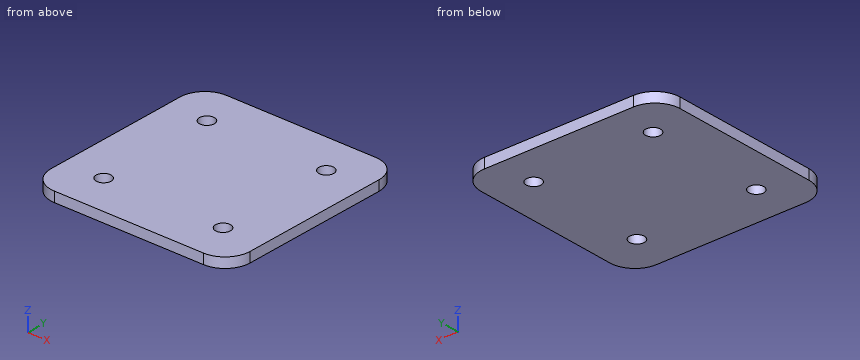
Autodesk Inventor part; units mm, degrees
ref_plane "YZ Plane" through (0, 0, 0) normal (1, 0, 0) x (0, 1, 0)
ref_plane "XZ Plane" through (0, 0, 0) normal (0, 1, 0) x (-1, 0, 0)
ref_plane "XY Plane" through (0, 0, 0) normal (0, 0, 1) x (1, 0, 0)
sketch "Sketch1" plane through (0, 0, 0) normal (0, 0, 1) x (1, 0, 0)
  line L0 (-20, -20) -> (20, -20)
  line L1 (20, -20) -> (20, 20)
  line L2 (20, 20) -> (-20, 20)
  line L3 (-20, 20) -> (-20, -20)
  line L4 (-20, -20) -> (20, 20) construction
  line L5 (20, -20) -> (-20, 20) construction
  line L6 (-12, -12) -> (12, -12) construction
  line L7 (12, -12) -> (12, 12) construction
  line L8 (12, 12) -> (-12, 12) construction
  line L9 (-12, 12) -> (-12, -12) construction
  line L10 (-12, -12) -> (12, 12) construction
  line L11 (12, -12) -> (-12, 12) construction
  point P0 (0, 0)
  dimension "d0" = 40
  dimension "d1" = 40
  dimension "d2" = 24
  dimension "d3" = 24
extrude "Extrusion1" add sketch "Sketch1" against normal blind 2
hole "Hole1" at (-12, 12, 0) at (12, 12, 0) at (12, -12, 0) at (-12, -12, 0) direction (0, 0, -1) diameter 3 depth 2
fillet "Fillet1" radius 5 4 edges at (20, 20, -1) (20, -20, -1) (-20, -20, -1) (-20, 20, -1)
properties part number "26" material "Gold"
Design review of the part built by this model. Coordinates are the model's own, in mm. Give positions to 0.01 mm unless a question says otherwise; leave off trailing zeros. Loops run counter-clockwise (first coordinate to the right, second up) from the corner with the lowest first, then second, coordinate; pieces in that order, holes last. Notation, with made-up numbers: M 15,80.25 L 40,80.25 A24 ccw 40,110.25 Z; hole C 73,79 d7. An arc over 180 degrees is marked long. One line per question, with ' | ' between items. Start each with the question number.
1. Add section A-A (z = -0.45). Write out the cut boundary in (x, y), plus the area to 3 significant figures.
2. To check wall thickness, follow L1, parallel to Y at x = -12, z = -1; L2, parallel to Y at x = -12.5, z = -1.15. State the ranges of each line that lie inside material, in increasing order.
3. Insertion check: P1, Ø2.5, axis at x = -12, y = -12, coming from the -Z side. The pin has a flat end and moves straight along its axis. Give the tip position at first contact, or say it passes through.
4. Add section B-B (x = -12). Write out the cut boundary in (y, z), plus the area to 3 significant figures.
Worked out:
1) outline: M -20,-15 A5 ccw -15,-20 L 15,-20 A5 ccw 20,-15 L 20,15 A5 ccw 15,20 L -15,20 A5 ccw -20,15 Z; hole C -12,-12 d3; hole C -12,12 d3; hole C 12,-12 d3; hole C 12,12 d3 | area: 1,550 mm²
2) L1: y = -20 to -13.5, -10.5 to 10.5, 13.5 to 20 | L2: y = -20 to -13.41, -10.59 to 10.59, 13.41 to 20
3) P1: passes through
4) outline: M -20,-2 L -13.5,-2 L -13.5,0 L -20,0 Z; M -10.5,-2 L 10.5,-2 L 10.5,0 L -10.5,0 Z; M 13.5,-2 L 20,-2 L 20,0 L 13.5,0 Z | area: 68.0 mm²
